Drawing for the job (mm, zero at the part's lowest x, y, z). A direction names the side the tool comes from. Give positions to 0.01 mm unless a question says otherwise; leave off trailing zeros. Order: outer loops, then holes, each group sorted by start corner. A loop starts at its lowest first (then second) coordinate and runs counter-clockwise, first axis right, second up. Notation, with made-up numbers: (88, 13.5) - (108, 13.5) arc R32 ccw to (108, 46.5) - close; hole circle Ø4 at (59.5, -10). An arc over 180 degrees is marked (long way). Use a Markdown table: item, result. Add a question column.
(1) Flat gauge pins, fed straight in: pin 1 (4 mm diameter, centred on x = 31, z = 7, fed in from +Y); pin 2 (1 mm diameter, centred on y = 32.5, z = 2.5, fed in from -X). Where does each tip first touch, or does it go through?
(2) Slice it at A-A (z = 7.75). Write the cut outline in (x, y), then the cut area to 3 significant figures.
(3) Which spindle directions (+Z, -Z, +X, -X, +Y, -Y) get a long thin tool onto all of the face, cutting with end or side? Do the marked faces 1, 2 and 3. Say none if no direction does.
(4) Slice it at C-C (y = 69). Write the cut outline in (x, z).
(5) Slice it at B-B (x = 57.5). Write the cut outline in (y, z), then the cut area to 3 significant figures.
(6) Wall check: line 1 (X direction, y = 39, z = 8); line 2 (Y direction, x = 21, z = 9). Give the ranges that are in metal, low to high.
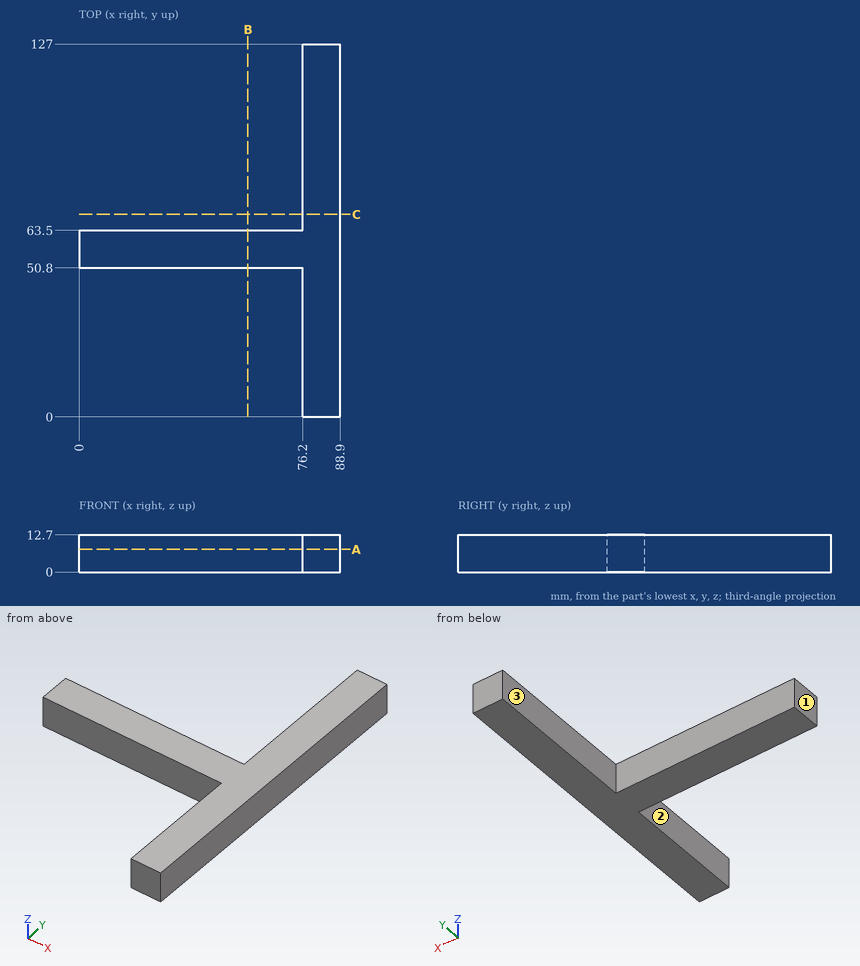
Solution:
| question | item | result |
|---|---|---|
| 1 | pin 1 | y = 63.5 |
| 1 | pin 2 | x = 76.2 |
| 2 | outline | (0, 50.8) - (76.2, 50.8) - (76.2, 0) - (88.9, 0) - (88.9, 127) - (76.2, 127) - (76.2, 63.5) - (0, 63.5) - close |
| 2 | area | 2,580 mm2 |
| 3 | face 1 | +Z, -Z, -X, +Y, -Y |
| 3 | face 2 | +Z, -Z, -X, -Y |
| 3 | face 3 | +Z, -Z, -X, +Y |
| 4 | outline | (76.2, 0) - (88.9, 0) - (88.9, 12.7) - (76.2, 12.7) - close |
| 5 | outline | (50.8, 0) - (63.5, 0) - (63.5, 12.7) - (50.8, 12.7) - close |
| 5 | area | 161 mm2 |
| 6 | line 1 | 76.2 to 88.9 |
| 6 | line 2 | 50.8 to 63.5 |
